Work out the finished part from the listing and answer in its coordinate system (mm). Face numbers are marked on the shaded views. A direction names the side the tool comes from. Give positions to 0.01 mm unless a question says otherwise; leave off trailing zeros. Loops run counter-clockwise (first coordinate to the right, second up) from the corner with the lowest first, then second, coordinate; pieces in that order, holes last. Notation, with made-up numbers: (26.25, 69.5) - (39.25, 69.5) arc R18 cw to (39.25, 80.5) - close; hole circle Ø10 at (-37.75, 19.25). An arc over 180 degrees is marked (long way). One line per question, with ' | ' between items. Start each with the question number.
1. Section C-C (y = -5.5) is taken. Determine the outline of the cut face in (x, z).
2. Section A-A (x = 0) is taken. Determine the outline of the cut face in (y, z), plus the area to 3 significant figures.
3. Section D-D (z = -2.25) is taken. Determine the outline of the cut face in (x, y).
4. Find the intervals of material crossed by line 1 (Z direction, x = 0, y = -4.75); line 2 (Y direction, x = -0.75, z = 6), in increasing order.
5. Section B-B (z = 7.75) is taken. Determine the outline of the cut face in (x, y).
6. For a pull along Y with two mould halves and no side action, classify the marked faces 3, 4, 5 and 6 as released by +Y, released by -Y, zero draft, split by the parting line, or undercut.
7. Which of the six approach directions +Z, -Z, +X, -X, +Y, -Y give full straight-line access (tool end or side, diameter ignored) to the marked faces 1 and 2?
8. This flat-tipped pin is pushed along its axis until it touches: pin 1 (4 mm diameter, centred on x = 0, z = -2.54, fed in from -Y). Where does it stop, or does it pass through?
from build123d import *

# Parameters (mm, degrees)
F0_W     = 20
F0_H     = 20
F0_W_2   = 15.2
F0_H_2   = 15.2
F1_DEPTH = 10
F2_T     = -2.4
F3_DEPTH = 6.2
F4_R     = 2.5
F5_DEPTH = 20.001
F6_R     = 1.2
F7_SIZE2 = 1
F7_SIZE  = 0.5


with BuildPart() as f1:
    # F0 (on Top) → F1 (new body)
    with BuildSketch(Plane.XY):
        Rectangle(F0_W, F0_H)
        Rectangle(F0_W_2, F0_H_2, mode=Mode.SUBTRACT)
        Rectangle(F0_W_2, F0_H_2)
    extrude(amount=F1_DEPTH)

    # F2
    f2_openings = [f1.faces().sort_by_distance(p)[0] for p in [
        (0, 0, 10),
    ]]
    offset(amount=F2_T, openings=f2_openings)

    # F3 (add): a face of the model
    f3_faces = [f1.faces().sort_by_distance(p)[0] for p in [
        (0, 0, 0),
    ]]
    extrude(f3_faces, amount=F3_DEPTH)

    # F4 (on face) → F5 (cut, through all)
    with BuildSketch(Plane(origin=(0, 10, 0), x_dir=(-1, 0, 0), z_dir=(0, 1, 0))):
        with Locations((0, -2.5408927461)):
            Circle(F4_R)
    extrude(amount=-F5_DEPTH, mode=Mode.SUBTRACT)

    # F6
    f6_edges = [f1.edges().sort_by_distance(p)[0] for p in [
        (-10, 10, 1.9),
        (10, 10, 1.9),
        (10, -10, 1.9),
        (-10, -10, 1.9),
    ]]
    fillet(f6_edges, radius=F6_R)

    # F7
    f7_edges = [f1.edges().sort_by_distance(p)[0] for p in [
        (10, 0, -6.2),
        (9.648528, -9.648528, -6.2),
        (9.648528, 9.648528, -6.2),
        (0, -10, -6.2),
        (0, 10, -6.2),
        (-9.648528, -9.648528, -6.2),
        (-9.648528, 9.648528, -6.2),
        (-10, 0, -6.2),
    ]]
    f7_side = f1.faces().sort_by_distance((0, 0, -6.2))[0]
    chamfer(f7_edges, length=F7_SIZE, length2=F7_SIZE2, reference=f7_side)


solid = f1.part
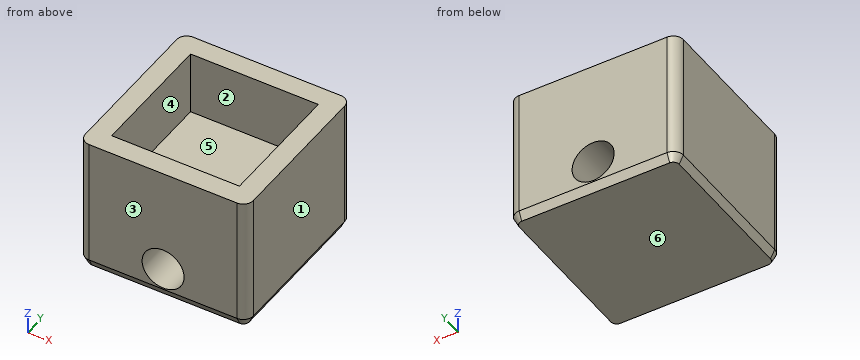
Conclusion:
1) outline: (-10, -5.2) - (-9.5, -6.2) - (9.5, -6.2) - (10, -5.2) - (10, 10) - (7.6, 10) - (7.6, 2.4) - (-7.6, 2.4) - (-7.6, 10) - (-10, 10) - close; hole circle Ø5 at (0, -2.54)
2) outline: (-10, -5.2) - (-9.5, -6.2) - (9.5, -6.2) - (10, -5.2) - (10, -5.04) - (-10, -5.04) - close; (-10, -0.04) - (10, -0.04) - (10, 10) - (7.6, 10) - (7.6, 2.4) - (-7.6, 2.4) - (-7.6, 10) - (-10, 10) - close | area: 108 mm²
3) outline: (-10, -8.8) arc R1.2 ccw to (-8.8, -10) - (-2.48, -10) - (-2.48, 10) - (-8.8, 10) arc R1.2 ccw to (-10, 8.8) - close; (2.48, -10) - (8.8, -10) arc R1.2 ccw to (10, -8.8) - (10, 8.8) arc R1.2 ccw to (8.8, 10) - (2.48, 10) - close
4) line 1: -6.2 to -5.04, -0.04 to 2.4 | line 2: -10 to -7.6, 7.6 to 10
5) outline: (-10, -8.8) arc R1.2 ccw to (-8.8, -10) - (8.8, -10) arc R1.2 ccw to (10, -8.8) - (10, 8.8) arc R1.2 ccw to (8.8, 10) - (-8.8, 10) arc R1.2 ccw to (-10, 8.8) - close; hole (-7.6, -7.6) - (7.6, -7.6) - (7.6, 7.6) - (-7.6, 7.6) - close
6) face 3: released by -Y | face 4: undercut | face 5: undercut | face 6: zero draft
7) face 1: +Z, -Z, +X, +Y, -Y | face 2: +Z
8) pin 1: through
